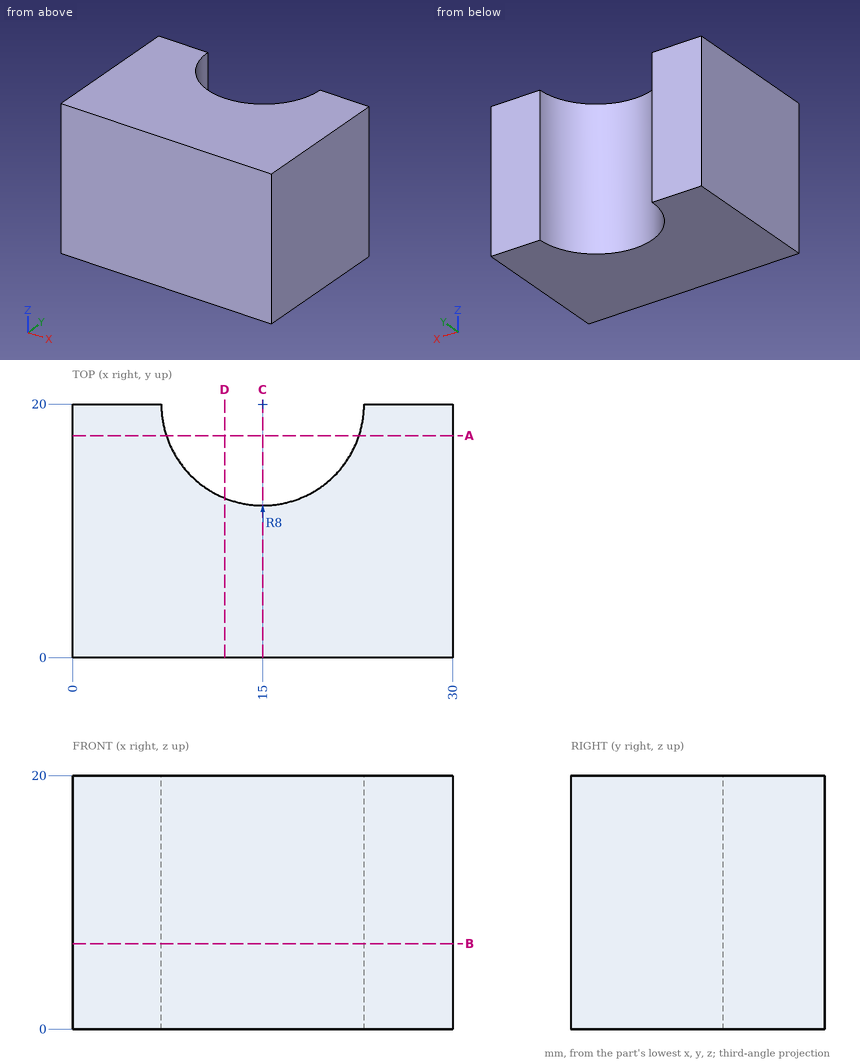
Can you work these out from the drawing? Everything is in mm from the part's minimum corner. Round coordinates to 2 decimals unless told otherwise and drop trailing zeros. Order: outer loops, then holes, each group sorted by start corner. A loop starts at its lowest first (then second) coordinate and runs counter-clockwise, first axis right, second up. Notation, with made-up numbers: (-37.5, 16) -> (-9.5, 16) arc R30 cw to (-9.5, 47) -> close; hole circle Ø6 at (-1.75, -35.5). An arc over 180 degrees is marked (long way). Use CSV: the item, a comma, the result in double quotes.
1. I want a section at A-A on y = 17.5. List the corners of the cut face in (x, z) for me.
Recorded:
outline,"(0, 0) -> (7.4, 0) -> (7.4, 20) -> (0, 20) -> close; (22.6, 0) -> (30, 0) -> (30, 20) -> (22.6, 20) -> close"
2. I need wall thicknesses on line 1 along X through (y, z) = (16, 4.5); line 2 along X through (y, z) = (16.5, 11); line 3 along Y through (x, z) = (16.75, 17.5). Which ranges of each line are inside material? Lowest first, please.
Recorded:
line 1,"x = 0 to 8.07, 21.93 to 30"
line 2,"x = 0 to 7.81, 22.19 to 30"
line 3,"y = 0 to 12.19"
3. I want a section at B-B on z = 6.75. List the corners of the cut face in (x, y) for me, and give its area (3 significant figures).
Recorded:
outline,"(0, 0) -> (30, 0) -> (30, 20) -> (23, 20) arc R8 cw to (7, 20) -> (0, 20) -> close"
area,"499 mm2"
4. I want a section at C-C on x = 15. List the corners of the cut face in (y, z) for me.
Recorded:
outline,"(0, 0) -> (12, 0) -> (12, 20) -> (0, 20) -> close"
5. I want a section at D-D on x = 12. List the corners of the cut face in (y, z) for me, and give its area (3 significant figures).
Recorded:
outline,"(0, 0) -> (12.58, 0) -> (12.58, 20) -> (0, 20) -> close"
area,"252 mm2"
